For this review, use the dimensioned drawing (mm, ordinates from the lowest corner) and the shaded views. A direction names the side the tool comes from. Coordinates: 2 decimals unless noted, no trailing zeros. Write each loop counter-clockwise with the first axis right and the second up, starting at its lowest first coordinate (ties: lowest second). Pieces come first, ordered by that corner, then holes. Notation, with made-up numbers: (-3.75, 81) - (8.25, 81) arc R30 cw to (8.25, 103) - close; hole circle Ø9 at (-39.5, -32). An arc over 180 degrees is marked (long way). One line per item, written item: value.
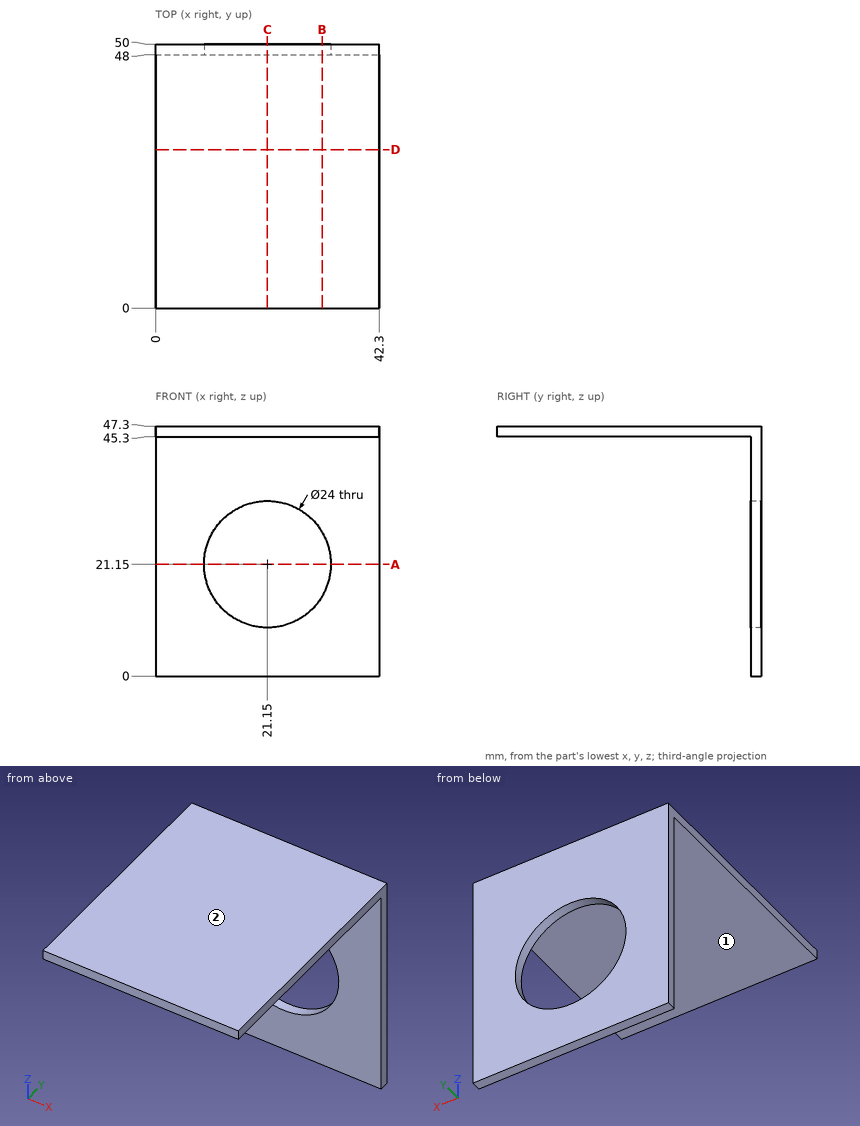
1. Consider section D-D, the plane y = 30. Write out the cut boundary in (x, z).
Answer block:
outline: (0, 45.3) - (42.3, 45.3) - (42.3, 47.3) - (0, 47.3) - close
2. Insertion check: pin 1 Ø10 at (x, y) = (19, 37) entering from -Z; pin 2 Ø21 at (x, z) = (12, 23.5) entering from -Y. Each pin has a flat end and moves straight along its axis. Give the tip position at first contact, or say it passes through.
Answer block:
pin 1: stops at z = 45.3
pin 2: stops at y = 48
3. Consider section B-B, the plane x = 31.5. Write out the cut boundary in (y, z).
Answer block:
outline: (0, 45.3) - (48, 45.3) - (48, 27.22) - (50, 27.22) - (50, 47.3) - (0, 47.3) - close; (48, 0) - (50, 0) - (50, 15.08) - (48, 15.08) - close
4. Wall thickness on line 1 along X through (y, z) = (48.8, 21.15); line 2 along Z through (x, y) = (21, 49); line 3 along Y through (x, z) = (8.5, 37): over which ranges is each line inside the solid? List them lowest first.
Answer block:
line 1: x = 0 to 9.15, 33.15 to 42.3
line 2: z = 0 to 9.15, 33.15 to 47.3
line 3: y = 48 to 50
5. Consider section A-A, the plane z = 21.15. Write out the cut boundary in (x, y), then the cut area to 3 significant figures.
Answer block:
outline: (0, 48) - (9.15, 48) - (9.15, 50) - (0, 50) - close; (33.15, 48) - (42.3, 48) - (42.3, 50) - (33.15, 50) - close
area: 36.6 mm^2
6. For the marked faces 1 and 2, list the 3-axis set-ups (+Z, -Z, +X, -X, +Y, -Y) from which the entire face can be reached by the end or side of a thin tool; tool diameter is ignored.
Answer block:
face 1: -Z, +X, -X, -Y
face 2: +Z, +X, -X, +Y, -Y
7. Consider section C-C, the plane x = 21.15. Write out the cut boundary in (y, z).
Answer block:
outline: (0, 45.3) - (48, 45.3) - (48, 33.15) - (50, 33.15) - (50, 47.3) - (0, 47.3) - close; (48, 0) - (50, 0) - (50, 9.15) - (48, 9.15) - close
